Verification items for the finished model (mm, model axes). Face numbers are marked on the shaded views. Coordinates: 2 decimals unless noted, no trailing zeros. Order: outer loops, then holes, each group sorted by start corner. A loop starts at its lowest first (then second) coordinate and runs counter-clockwise, first axis right, second up. Notation, with made-up numbers: (54, 0.5) -> (85, 0.5) arc R28 cw to (85, 35.5) -> close; hole circle Ø2 at (-7.75, 71.25). An arc over 180 degrees is marked (long way). Write item = value, one per line. Start each with the question number.
from build123d import *

# Parameters (mm, degrees)
SKETCH1_W           = 500
SKETCH1_H           = 450
SKETCH1_W_2         = 390
SKETCH1_H_2         = 285
BOSS_EXTRUDE1_DEPTH = 19
SKETCH2_W           = 12
SKETCH2_H           = 438
BOSS_EXTRUDE4_DEPTH = 18
SKETCH3_W           = 500
SKETCH3_H           = 12
BOSS_EXTRUDE5_DEPTH = 18
SKETCH4_W           = 12
SKETCH4_H           = 438
BOSS_EXTRUDE6_DEPTH = 18


with BuildPart() as part:
    # Sketch1 → Boss-Extrude1 (new body)
    with BuildSketch(Plane(origin=(0, 0, 0), x_dir=(0, 0, -1), z_dir=(1, 0, 0))):
        with Locations((250, 225)):
            Rectangle(SKETCH1_W, SKETCH1_H)
        with Locations((250, 217.5)):
            Rectangle(SKETCH1_W_2, SKETCH1_H_2, mode=Mode.SUBTRACT)
    extrude(amount=BOSS_EXTRUDE1_DEPTH)

    # Sketch2 → Boss-Extrude4 (add)
    with BuildSketch(Plane(origin=(19, 0, 0), x_dir=(0, 0, -1), z_dir=(1, 0, 0))):
        with Locations((6, 219)):
            Rectangle(SKETCH2_W, SKETCH2_H)
    extrude(amount=BOSS_EXTRUDE4_DEPTH)

    # Sketch3 → Boss-Extrude5 (add)
    with BuildSketch(Plane(origin=(19, 0, 0), x_dir=(0, 0, -1), z_dir=(1, 0, 0))):
        with Locations((250, 444)):
            Rectangle(SKETCH3_W, SKETCH3_H)
    extrude(amount=BOSS_EXTRUDE5_DEPTH)

    # Sketch4 → Boss-Extrude6 (add)
    with BuildSketch(Plane(origin=(19, 0, 0), x_dir=(0, 0, -1), z_dir=(1, 0, 0))):
        with Locations((494, 219)):
            Rectangle(SKETCH4_W, SKETCH4_H)
    extrude(amount=BOSS_EXTRUDE6_DEPTH)


solid = part.part
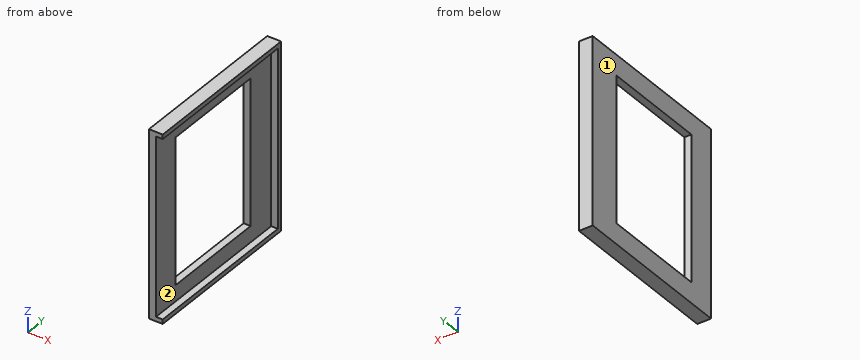
Item 1: Section check C-C (x = 12.5). Record the boundary of the cut face in (y, z).
Item 2: Gauge pin test, flat ends, axial feed: P1, Ø9.5, axis at x = 9, y = 215.5, coming from the +Z side; P2, Ø2, axis at x = 21, z = -283, coming from the -Y side. Record the tip position at first contact, or that the pin passes through.
Item 3: Thickness scan on line 1 (Z direction, x = 2, y = 269); line 2 (Z direction, x = 33, y = 180.5); line 3 (Y direction, x = 17.5, z = -114). Record the ranges inside material, lowest first.
Item 4: Section check B-B (y = 335). Record the boundary of the cut face in (x, z), then the cut area to 3 significant figures.
Item 5: Section check A-A (z = -355). Record the boundary of the cut face in (x, y).
Item 6: Mould release check, pull along Z, two halves, no side actions. Record for the marked faces 1 and 2: pulls with the +Z half, pulls with the -Z half, needs draft (parallel to the pull), parting line crosses it, or undercut.
Item 7: Section check D-D (z = -46.5). Record the boundary of the cut face in (x, y).
Filled sheet:
q1.outline = (0, -500) -> (450, -500) -> (450, 0) -> (0, 0) -> close; hole (75, -445) -> (360, -445) -> (360, -55) -> (75, -55) -> close
q2.P1 = 0
q2.P2 = 438
q3.line_1 = -500 to -445, -55 to 0
q3.line_2 = -500 to -488, -12 to 0
q3.line_3 = 0 to 75, 360 to 450
q4.outline = (0, -500) -> (37, -500) -> (37, -488) -> (19, -488) -> (19, -445) -> (0, -445) -> close; (0, -55) -> (19, -55) -> (19, -12) -> (37, -12) -> (37, 0) -> (0, 0) -> close
q4.area = 2,520 mm^2
q5.outline = (0, 0) -> (19, 0) -> (19, 75) -> (0, 75) -> close; (0, 360) -> (19, 360) -> (19, 438) -> (37, 438) -> (37, 450) -> (0, 450) -> close
q6.face_1 = needs draft
q6.face_2 = undercut
q7.outline = (0, 0) -> (19, 0) -> (19, 438) -> (37, 438) -> (37, 450) -> (0, 450) -> close
